from build123d import *

# Parameters (mm, degrees)
ESQUISSE1_W             = 17.78
ESQUISSE1_H             = 20.955
ESQUISSE1_R             = 0.425
BOSS_EXTRU_1_DEPTH      = 2
BOSS_EXTRU_2_DEPTH      = 2
CONG_1_R                = 1
ESQUISSE3_W             = 6.499332414
ESQUISSE3_H             = 0.15
ENL_V_MAT_EXTRU_1_DEPTH = 4
CONG_2_R                = 1
ESQUISSE4_W             = 12.79
ESQUISSE4_H             = 10.16
BOSS_EXTRU_3_DEPTH      = 2
ESQUISSE5_W             = 4
ESQUISSE5_H             = 2
ESQUISSE5_W_2           = 1.5
ESQUISSE5_H_2           = 1.5
BOSS_EXTRU_4_DEPTH      = 0.5
ESQUISSE6_R             = 0.75
BOSS_EXTRU_5_DEPTH      = 0.5


with BuildPart() as part:
    # Esquisse1 → Boss.-Extru.1 (new body)
    with BuildSketch(Plane(origin=(0, 0, 0), x_dir=(1, 0, 0), z_dir=(0, 1, 0))):
        Rectangle(ESQUISSE1_W, ESQUISSE1_H)
        with Locations(Location((-7.56, 7.4775, 0), (0, 0, 270))):
            Circle(ESQUISSE1_R, mode=Mode.SUBTRACT)
        with Locations(Location((7.68, 7.4775, 0), (0, 0, 270))):
            Circle(ESQUISSE1_R, mode=Mode.SUBTRACT)
        with Locations(Location((7.68, 4.9375, 0), (0, 0, 270))):
            Circle(ESQUISSE1_R, mode=Mode.SUBTRACT)
        with Locations(Location((7.68, 2.3975, 0), (0, 0, 270))):
            Circle(ESQUISSE1_R, mode=Mode.SUBTRACT)
        with Locations(Location((7.68, -0.1425, 0), (0, 0, 270))):
            Circle(ESQUISSE1_R, mode=Mode.SUBTRACT)
        with Locations(Location((7.68, -2.6825, 0), (0, 0, 270))):
            Circle(ESQUISSE1_R, mode=Mode.SUBTRACT)
        with Locations(Location((7.68, -5.2225, 0), (0, 0, 270))):
            Circle(ESQUISSE1_R, mode=Mode.SUBTRACT)
        with Locations(Location((7.68, -7.7625, 0), (0, 0, 270))):
            Circle(ESQUISSE1_R, mode=Mode.SUBTRACT)
        with Locations(Location((-7.56, 4.9375, 0), (0, 0, 270))):
            Circle(ESQUISSE1_R, mode=Mode.SUBTRACT)
        with Locations(Location((-7.56, 2.3975, 0), (0, 0, 270))):
            Circle(ESQUISSE1_R, mode=Mode.SUBTRACT)
        with Locations(Location((-7.56, -0.1425, 0), (0, 0, 270))):
            Circle(ESQUISSE1_R, mode=Mode.SUBTRACT)
        with Locations(Location((-7.56, -2.6825, 0), (0, 0, 270))):
            Circle(ESQUISSE1_R, mode=Mode.SUBTRACT)
        with Locations(Location((-7.56, -5.2225, 0), (0, 0, 270))):
            Circle(ESQUISSE1_R, mode=Mode.SUBTRACT)
        with Locations(Location((-7.56, -7.7625, 0), (0, 0, 270))):
            Circle(ESQUISSE1_R, mode=Mode.SUBTRACT)
    extrude(amount=BOSS_EXTRU_1_DEPTH)

    # Esquisse2 → Boss.-Extru.2 (add)
    with BuildSketch(Plane(origin=(0, 2, 0), x_dir=(1, 0, 0), z_dir=(0, 1, 0))):
        Polygon((-4.5, 12.0175), (4.5, 12.0175), (4.5, 7.4775), (4.5, 4.9375), (-4.5, 4.9375), (-4.5, 7.4775), align=None)
    extrude(amount=BOSS_EXTRU_2_DEPTH)

    # Congé1
    cong_1_edges = [part.edges().sort_by_distance(p)[0] for p in [
        (-4.5, 2, -11.2475),
        (4.5, 2, -11.2475),
        (-4.5, 4, -8.4775),
        (4.5, 4, -8.4775),
    ]]
    fillet(cong_1_edges, radius=CONG_1_R - 0.0001)  # a hair under: the kernel refuses the full size

    # Esquisse3 → Enlèv. mat.-Extru.1 (cut)
    with BuildSketch(Plane(origin=(0, 0, -12.0175), x_dir=(-1, 0, 0), z_dir=(0, 0, -1))):
        with BuildLine():
            ThreePointArc((-3.708196785, 2.958530578), (-3.568140241, 2.640056544), (-3.249666207, 2.5))
            Line((-3.249666207, 2.5), (3.249666207, 2.5))
            ThreePointArc((3.249666207, 2.5), (3.568140241, 2.640056544), (3.708196785, 2.958530578))
            Line((3.708196785, 2.958530578), (3.708196785, 3))
            Line((3.708196785, 3), (3.708196785, 3.041469422))
            ThreePointArc((3.708196785, 3.041469422), (3.568140241, 3.359943456), (3.249666207, 3.5))
            Line((3.249666207, 3.5), (-3.249666207, 3.5))
            ThreePointArc((-3.249666207, 3.5), (-3.568140241, 3.359943456), (-3.708196785, 3.041469422))
            Line((-3.708196785, 3.041469422), (-3.708196785, 3))
            Line((-3.708196785, 3), (-3.708196785, 2.958530578))
        make_face()
        with Locations((0, 3)):
            Rectangle(ESQUISSE3_W, ESQUISSE3_H, mode=Mode.SUBTRACT)
    extrude(amount=-ENL_V_MAT_EXTRU_1_DEPTH, mode=Mode.SUBTRACT)

    # Congé2
    cong_2_edges = [part.edges().sort_by_distance(p)[0] for p in [
        (8.89, 1, 10.4775),
        (-8.89, 1, 10.4775),
        (-8.89, 1, -10.4775),
        (8.89, 1, -10.4775),
    ]]
    fillet(cong_2_edges, radius=CONG_2_R)

    # Esquisse4 → Boss.-Extru.3 (add)
    with BuildSketch(Plane(origin=(0, 2, 0), x_dir=(1, 0, 0), z_dir=(0, 1, 0))):
        with Locations((0.06, -1.4125)):
            Rectangle(ESQUISSE4_W, ESQUISSE4_H)
    extrude(amount=BOSS_EXTRU_3_DEPTH)

    # Esquisse5 → Boss.-Extru.4 (add)
    with BuildSketch(Plane(origin=(0, 2, 0), x_dir=(1, 0, 0), z_dir=(0, 1, 0))):
        with Locations((-4.125, -8.44125)):
            Rectangle(ESQUISSE5_W, ESQUISSE5_H)
        with Locations((4.245, -8.44125)):
            Rectangle(ESQUISSE5_W, ESQUISSE5_H)
        with Locations((0.06, -8.44125)):
            Rectangle(ESQUISSE5_W_2, ESQUISSE5_H_2)
    extrude(amount=BOSS_EXTRU_4_DEPTH)

    # Esquisse6 → Boss.-Extru.5 (add)
    with BuildSketch(Plane(origin=(0, 2.5, 0), x_dir=(1, 0, 0), z_dir=(0, 1, 0))):
        with Locations(Location((-4.125, -8.44125, 0), (0, 0, 270))):
            Circle(ESQUISSE6_R)
        with Locations(Location((4.245, -8.44125, 0), (0, 0, 90))):
            Circle(ESQUISSE6_R)
    extrude(amount=BOSS_EXTRU_5_DEPTH)


solid = part.part
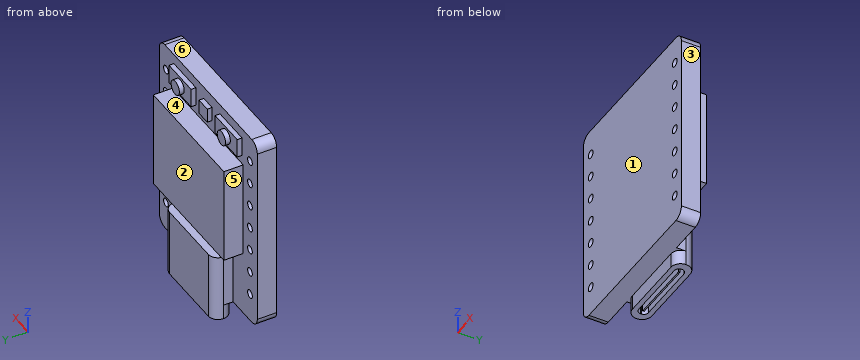
Geometry check sheet. Reference: the model listing, model coordinates, mm. Face numbers are marked on the shaded views. A direction names the side the tool comes from. Round coordinates to 2 decimals unless told otherwise and drop trailing zeros. Write each loop counter-clockwise with the first axis right and the second up, starting at its lowest first coordinate (ties: lowest second). Pieces come first, ordered by that corner, then holes. Notation, with made-up numbers: (5, -32) - (22, -32) arc R28 cw to (22, -2) - close; hole circle Ø6 at (76, -16.75). An arc over 180 degrees is marked (long way). One line per item, written item: value.
1. Depth check by flat-ended pin: pin 1 Ø1 at (x, y) = (-2.5, 3.5) entering from +Z; pin 2 Ø0.8 at (x, z) = (-4.5, 8.5) entering from +Y; pin 3 Ø1.2 at (x, z) = (0, 8) entering from +Y. Enter the tip coordinate at first touch or a pass-through.
The answers:
pin 1: stops at z = 6.49
pin 2: stops at y = 3
pin 3: stops at y = 2.5
2. Scan lines: L1, parallel to Y at x = -2.75, z = -9 (3 decimals); L2, parallel to X at y = 1, z = -7.5; L3, parallel to Y at x = 3, z = -11 (3 decimals). Record each from-to range of solid material in increasing order.
The answers:
L1: y = 0 to 2.5, 2.925 to 3.075, 3.5 to 4
L2: x = -8.89 to -7.98, -7.14 to 7.26, 8.1 to 8.89
L3: y = 2 to 2.5, 2.925 to 3.075, 3.5 to 4
3. Cross-section at A-A on x = -7.56. Give the number of separate pieces and of enclosed holes in the cut face, and give its area (3 significant figures).
The answers:
separate pieces: 8
enclosed holes: 0
area: 30.0 mm^2
4. Cross-section at C-C on z = 6. Record the boundary of the cut face in (x, y) (3 decimals).
The answers:
outline: (-8.89, 0) - (8.89, 0) - (8.89, 2) - (6.455, 2) - (6.455, 4) - (-6.335, 4) - (-6.335, 2) - (-8.89, 2) - close
5. Set-up check for the marked faces 4, 5 and 6: record each of +Z, -Z, +X, -X, +Y, -Y from which the full face is reachable in a straight line by a thin tool's end or side.
The answers:
face 4: +X, -X, +Y
face 5: +Z, -Z, -X, +Y
face 6: +Z, +X, -X, +Y, -Y
6. Mould release check, pull along Y, two halves, no side actions. Record for the marked faces 1, 2 and 3: released by +Y, released by -Y, zero draft, split by the parting line, or undercut.
The answers:
face 1: released by -Y
face 2: released by +Y
face 3: zero draft
